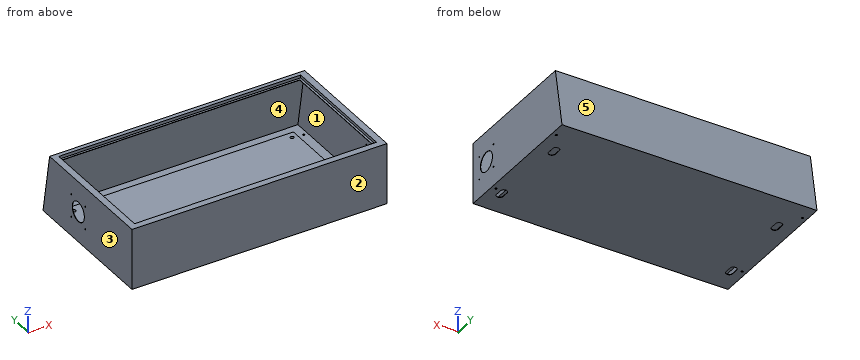
from build123d import *

# Parameters (mm, degrees)
SKETCH_1_W          = 1170
SKETCH_1_H          = 663
EXTRUDE_1_DEPTH     = 280
SKETCH_2_W          = 1110
SKETCH_2_H          = 564.628445402
CUT_EXTRUDE_1_DEPTH = 13.5
SKETCH_4_W          = 1090
SKETCH_4_H          = 544.628445402
CUT_EXTRUDE_2_DEPTH = 1.5
SHELL_START         = -583.5
SHELL_1_DEPTH       = 1167
SHELL_1_2_OUTLINE_W = 567.628445402
SHELL_1_2_OUTLINE_H = 13.5
SHELL_1_2_DEPTH     = 27
SHELL_START_2       = 556.5
SHELL_1_3_OUTLINE_W = 567.628445402
SHELL_1_3_OUTLINE_H = 13.5
SHELL_1_3_DEPTH     = 27
CUT_EXTRUDE_3_REACH = 730.366
SKETCH_5_R          = 4.5
CUT_EXTRUDE_4_REACH = 1249.875
SKETCH_6_R          = 45
SKETCH_6_R_2        = 2.75
CUT_EXTRUDE_6_REACH = 1249.875
SKETCH_8_R          = 45
SKETCH_8_R_2        = 2.75
SKETCH_9_W          = 1050
SKETCH_9_H          = 590
EXTRUDE_2_DEPTH     = 20
SKETCH_10_R         = 8.286870523
CUT_EXTRUDE_7_DEPTH = 10


# Read off the part's stored shape, not the designer's step: 抽壳1
with BuildPart() as part:
    # 草图1 → 凸台-拉伸1 (new body)
    with BuildSketch(Plane.XY):
        Rectangle(SKETCH_1_W, SKETCH_1_H)
    extrude(amount=EXTRUDE_1_DEPTH)

    # Split Bodies 1
    split(bisect_by=Plane(origin=(0, 321.504051895, 56.689838756), x_dir=(0, -0.17364817766691376, 0.984807753012211), z_dir=(0, 0.984807753012211, 0.17364817766691376)), keep=Keep.BOTTOM)

    # 草图2 → 切除-拉伸1 (cut)
    with BuildSketch(Plane.XY.offset(280)):
        with Locations((0, -19.185777299)):
            Rectangle(SKETCH_2_W, SKETCH_2_H)
    extrude(amount=-CUT_EXTRUDE_1_DEPTH, mode=Mode.SUBTRACT)

    # 草图4 → 切除-拉伸2 (cut)
    with BuildSketch(Plane.XY.offset(266.5)):
        with Locations((0, -19.185777299)):
            Rectangle(SKETCH_4_W, SKETCH_4_H)
    extrude(amount=-CUT_EXTRUDE_2_DEPTH, mode=Mode.SUBTRACT)

    # 抽壳1 outline → 抽壳1 (cut)
    with BuildSketch(Plane.YZ.offset(SHELL_START)):
        Polygon((-330, 1.5), (329.712369611, 1.5), (280.869795955, 278.5), (264.628445402, 278.5), (264.628445402, 265), (-303, 265), (-303, 278.5), (-330, 278.5), align=None)
    extrude(amount=SHELL_1_DEPTH, mode=Mode.SUBTRACT)

    # Shell 1 2 outline → Shell 1 2 (cut)
    with BuildSketch(Plane.YZ.offset(SHELL_START)):
        with Locations((-19.185777299, 271.75)):
            Rectangle(SHELL_1_2_OUTLINE_W, SHELL_1_2_OUTLINE_H)
    extrude(amount=SHELL_1_2_DEPTH, mode=Mode.SUBTRACT)

    # Shell 1 3 outline → Shell 1 3 (cut)
    with BuildSketch(Plane.YZ.offset(SHELL_START_2)):
        with Locations((-19.185777299, 271.75)):
            Rectangle(SHELL_1_3_OUTLINE_W, SHELL_1_3_OUTLINE_H)
    extrude(amount=SHELL_1_3_DEPTH, mode=Mode.SUBTRACT)

    # 草图5 → 切除-拉伸3 (cut, up to next)
    with BuildSketch(Plane(origin=(0, 0, 0), x_dir=(-1, 0, 0), z_dir=(0, 0, -1)), mode=Mode.PRIVATE) as cut_extrude_3_sk1:
        with Locations((-565, 256.5)):
            Circle(SKETCH_5_R)
    cut_extrude_3_tool1 = extrude(cut_extrude_3_sk1.sketch, amount=-CUT_EXTRUDE_3_REACH, mode=Mode.PRIVATE) & part.part
    # 草图5 → 切除-拉伸3 (cut, up to next)
    with BuildSketch(Plane(origin=(0, 0, 0), x_dir=(-1, 0, 0), z_dir=(0, 0, -1)), mode=Mode.PRIVATE) as cut_extrude_3_sk2:
        with Locations((-565, -193.5)):
            Circle(SKETCH_5_R)
    cut_extrude_3_tool2 = extrude(cut_extrude_3_sk2.sketch, amount=-CUT_EXTRUDE_3_REACH, mode=Mode.PRIVATE) & part.part
    # 草图5 → 切除-拉伸3 (cut, up to next)
    with BuildSketch(Plane(origin=(0, 0, 0), x_dir=(-1, 0, 0), z_dir=(0, 0, -1)), mode=Mode.PRIVATE) as cut_extrude_3_sk3:
        with Locations(Location((565, 256.5, 0), (0, 0, 180))):
            Circle(SKETCH_5_R)
    cut_extrude_3_tool3 = extrude(cut_extrude_3_sk3.sketch, amount=-CUT_EXTRUDE_3_REACH, mode=Mode.PRIVATE) & part.part
    # 草图5 → 切除-拉伸3 (cut, up to next)
    with BuildSketch(Plane(origin=(0, 0, 0), x_dir=(-1, 0, 0), z_dir=(0, 0, -1)), mode=Mode.PRIVATE) as cut_extrude_3_sk4:
        with Locations(Location((565, -193.5, 0), (0, 0, 180))):
            Circle(SKETCH_5_R)
    cut_extrude_3_tool4 = extrude(cut_extrude_3_sk4.sketch, amount=-CUT_EXTRUDE_3_REACH, mode=Mode.PRIVATE) & part.part
    # 草图5 → 切除-拉伸3 (cut, up to next)
    with BuildSketch(Plane(origin=(0, 0, 0), x_dir=(-1, 0, 0), z_dir=(0, 0, -1)), mode=Mode.PRIVATE) as cut_extrude_3_sk5:
        with BuildLine():
            Line((511.5, -196.5), (511.5, -226.5))
            ThreePointArc((511.5, -226.5), (526.5, -241.5), (541.5, -226.5))
            Line((541.5, -226.5), (541.5, -196.5))
            ThreePointArc((541.5, -196.5), (526.5, -181.5), (511.5, -196.5))
        make_face()
    cut_extrude_3_tool5 = extrude(cut_extrude_3_sk5.sketch, amount=-CUT_EXTRUDE_3_REACH, mode=Mode.PRIVATE) & part.part
    # 草图5 → 切除-拉伸3 (cut, up to next)
    with BuildSketch(Plane(origin=(0, 0, 0), x_dir=(-1, 0, 0), z_dir=(0, 0, -1)), mode=Mode.PRIVATE) as cut_extrude_3_sk6:
        with BuildLine():
            Line((526.5, 167.237), (526.5, 137.237))
            ThreePointArc((526.5, 137.237), (511.5, 122.237), (496.5, 137.237))
            Line((496.5, 137.237), (496.5, 167.237))
            ThreePointArc((496.5, 167.237), (511.5, 182.237), (526.5, 167.237))
        make_face()
    cut_extrude_3_tool6 = extrude(cut_extrude_3_sk6.sketch, amount=-CUT_EXTRUDE_3_REACH, mode=Mode.PRIVATE) & part.part
    # 草图5 → 切除-拉伸3 (cut, up to next)
    with BuildSketch(Plane(origin=(0, 0, 0), x_dir=(-1, 0, 0), z_dir=(0, 0, -1)), mode=Mode.PRIVATE) as cut_extrude_3_sk7:
        with BuildLine():
            Line((-541.5, -196.5), (-541.5, -226.5))
            ThreePointArc((-541.5, -226.5), (-526.5, -241.5), (-511.5, -226.5))
            Line((-511.5, -226.5), (-511.5, -196.5))
            ThreePointArc((-511.5, -196.5), (-526.5, -181.5), (-541.5, -196.5))
        make_face()
    cut_extrude_3_tool7 = extrude(cut_extrude_3_sk7.sketch, amount=-CUT_EXTRUDE_3_REACH, mode=Mode.PRIVATE) & part.part
    # 草图5 → 切除-拉伸3 (cut, up to next)
    with BuildSketch(Plane(origin=(0, 0, 0), x_dir=(-1, 0, 0), z_dir=(0, 0, -1)), mode=Mode.PRIVATE) as cut_extrude_3_sk8:
        with BuildLine():
            Line((-496.5, 167.237), (-496.5, 137.237))
            ThreePointArc((-496.5, 137.237), (-511.5, 122.237), (-526.5, 137.237))
            Line((-526.5, 137.237), (-526.5, 167.237))
            ThreePointArc((-526.5, 167.237), (-511.5, 182.237), (-496.5, 167.237))
        make_face()
    cut_extrude_3_tool8 = extrude(cut_extrude_3_sk8.sketch, amount=-CUT_EXTRUDE_3_REACH, mode=Mode.PRIVATE) & part.part
    add(cut_extrude_3_tool1.solids().sort_by_distance((565, 256.5, 0))[0], mode=Mode.SUBTRACT)
    add(cut_extrude_3_tool2.solids().sort_by_distance((565, -193.5, 0))[0], mode=Mode.SUBTRACT)
    add(cut_extrude_3_tool3.solids().sort_by_distance((-565, 256.5, 0))[0], mode=Mode.SUBTRACT)
    add(cut_extrude_3_tool4.solids().sort_by_distance((-565, -193.5, 0))[0], mode=Mode.SUBTRACT)
    add(cut_extrude_3_tool5.solids().sort_by_distance((-526.5, -211.5, 0))[0], mode=Mode.SUBTRACT)
    add(cut_extrude_3_tool6.solids().sort_by_distance((-511.5, 152.237, 0))[0], mode=Mode.SUBTRACT)
    add(cut_extrude_3_tool7.solids().sort_by_distance((526.5, -211.5, 0))[0], mode=Mode.SUBTRACT)
    add(cut_extrude_3_tool8.solids().sort_by_distance((511.5, 152.237, 0))[0], mode=Mode.SUBTRACT)

    # 草图6 → 切除-拉伸4 (cut, up to next)
    with BuildSketch(Plane(origin=(585, 0, 0), x_dir=(0, 0, -1), z_dir=(1, 0, 0)), mode=Mode.PRIVATE) as cut_extrude_4_sk1:
        with Locations((-140, -231.5)):
            Circle(SKETCH_6_R)
    cut_extrude_4_tool1 = extrude(cut_extrude_4_sk1.sketch, amount=-CUT_EXTRUDE_4_REACH, mode=Mode.PRIVATE) & part.part
    # 草图6 → 切除-拉伸4 (cut, up to next)
    with BuildSketch(Plane(origin=(585, 0, 0), x_dir=(0, 0, -1), z_dir=(1, 0, 0)), mode=Mode.PRIVATE) as cut_extrude_4_sk2:
        with Locations((-87.5, -179)):
            Circle(SKETCH_6_R_2)
    cut_extrude_4_tool2 = extrude(cut_extrude_4_sk2.sketch, amount=-CUT_EXTRUDE_4_REACH, mode=Mode.PRIVATE) & part.part
    # 草图6 → 切除-拉伸4 (cut, up to next)
    with BuildSketch(Plane(origin=(585, 0, 0), x_dir=(0, 0, -1), z_dir=(1, 0, 0)), mode=Mode.PRIVATE) as cut_extrude_4_sk3:
        with Locations(Location((-192.5, -179, 0), (0, 0, 180))):
            Circle(SKETCH_6_R_2)
    cut_extrude_4_tool3 = extrude(cut_extrude_4_sk3.sketch, amount=-CUT_EXTRUDE_4_REACH, mode=Mode.PRIVATE) & part.part
    # 草图6 → 切除-拉伸4 (cut, up to next)
    with BuildSketch(Plane(origin=(585, 0, 0), x_dir=(0, 0, -1), z_dir=(1, 0, 0)), mode=Mode.PRIVATE) as cut_extrude_4_sk4:
        with Locations((-192.5, -284)):
            Circle(SKETCH_6_R_2)
    cut_extrude_4_tool4 = extrude(cut_extrude_4_sk4.sketch, amount=-CUT_EXTRUDE_4_REACH, mode=Mode.PRIVATE) & part.part
    # 草图6 → 切除-拉伸4 (cut, up to next)
    with BuildSketch(Plane(origin=(585, 0, 0), x_dir=(0, 0, -1), z_dir=(1, 0, 0)), mode=Mode.PRIVATE) as cut_extrude_4_sk5:
        with Locations(Location((-87.5, -284, 0), (0, 0, 180))):
            Circle(SKETCH_6_R_2)
    cut_extrude_4_tool5 = extrude(cut_extrude_4_sk5.sketch, amount=-CUT_EXTRUDE_4_REACH, mode=Mode.PRIVATE) & part.part
    add(cut_extrude_4_tool1.solids().sort_by_distance((585, -231.5, 140))[0], mode=Mode.SUBTRACT)
    add(cut_extrude_4_tool2.solids().sort_by_distance((585, -179, 87.5))[0], mode=Mode.SUBTRACT)
    add(cut_extrude_4_tool3.solids().sort_by_distance((585, -179, 192.5))[0], mode=Mode.SUBTRACT)
    add(cut_extrude_4_tool4.solids().sort_by_distance((585, -284, 192.5))[0], mode=Mode.SUBTRACT)
    add(cut_extrude_4_tool5.solids().sort_by_distance((585, -284, 87.5))[0], mode=Mode.SUBTRACT)

    # 草图8 → 切除-拉伸6 (cut, up to next)
    with BuildSketch(Plane.ZY.offset(585), mode=Mode.PRIVATE) as cut_extrude_6_sk1:
        with Locations((140, 68.5)):
            Circle(SKETCH_8_R)
    cut_extrude_6_tool1 = extrude(cut_extrude_6_sk1.sketch, amount=-CUT_EXTRUDE_6_REACH, mode=Mode.PRIVATE) & part.part
    # 草图8 → 切除-拉伸6 (cut, up to next)
    with BuildSketch(Plane.ZY.offset(585), mode=Mode.PRIVATE) as cut_extrude_6_sk2:
        with Locations((192.5, 16)):
            Circle(SKETCH_8_R_2)
    cut_extrude_6_tool2 = extrude(cut_extrude_6_sk2.sketch, amount=-CUT_EXTRUDE_6_REACH, mode=Mode.PRIVATE) & part.part
    # 草图8 → 切除-拉伸6 (cut, up to next)
    with BuildSketch(Plane.ZY.offset(585), mode=Mode.PRIVATE) as cut_extrude_6_sk3:
        with Locations((87.5, 16)):
            Circle(SKETCH_8_R_2)
    cut_extrude_6_tool3 = extrude(cut_extrude_6_sk3.sketch, amount=-CUT_EXTRUDE_6_REACH, mode=Mode.PRIVATE) & part.part
    # 草图8 → 切除-拉伸6 (cut, up to next)
    with BuildSketch(Plane.ZY.offset(585), mode=Mode.PRIVATE) as cut_extrude_6_sk4:
        with Locations((87.5, 121)):
            Circle(SKETCH_8_R_2)
    cut_extrude_6_tool4 = extrude(cut_extrude_6_sk4.sketch, amount=-CUT_EXTRUDE_6_REACH, mode=Mode.PRIVATE) & part.part
    # 草图8 → 切除-拉伸6 (cut, up to next)
    with BuildSketch(Plane.ZY.offset(585), mode=Mode.PRIVATE) as cut_extrude_6_sk5:
        with Locations((192.5, 121)):
            Circle(SKETCH_8_R_2)
    cut_extrude_6_tool5 = extrude(cut_extrude_6_sk5.sketch, amount=-CUT_EXTRUDE_6_REACH, mode=Mode.PRIVATE) & part.part
    add(cut_extrude_6_tool1.solids().sort_by_distance((-585, 68.5, 140))[0], mode=Mode.SUBTRACT)
    add(cut_extrude_6_tool2.solids().sort_by_distance((-585, 16, 192.5))[0], mode=Mode.SUBTRACT)
    add(cut_extrude_6_tool3.solids().sort_by_distance((-585, 16, 87.5))[0], mode=Mode.SUBTRACT)
    add(cut_extrude_6_tool4.solids().sort_by_distance((-585, 121, 87.5))[0], mode=Mode.SUBTRACT)
    add(cut_extrude_6_tool5.solids().sort_by_distance((-585, 121, 192.5))[0], mode=Mode.SUBTRACT)

    # 草图9 → 凸台-拉伸2 (add)
    with BuildSketch(Plane.XY.offset(1.5)):
        with Locations((0, -26.5)):
            Rectangle(SKETCH_9_W, SKETCH_9_H)
    extrude(amount=EXTRUDE_2_DEPTH)

    # 草图10 → 切除-拉伸7 (cut)
    with BuildSketch(Plane.XY.offset(21.5)):
        with Locations((-500.232706652, 237.876964373)):
            Circle(SKETCH_10_R)
        with Locations(Location((500.232706652, 237.876964373, 0), (0, 0, 180))):
            Circle(SKETCH_10_R)
        with Locations((500.232706652, -288.753501232)):
            Circle(SKETCH_10_R)
        with Locations(Location((-500.232706652, -288.753501232, 0), (0, 0, 180))):
            Circle(SKETCH_10_R)
    extrude(amount=-CUT_EXTRUDE_7_DEPTH, mode=Mode.SUBTRACT)


solid = part.part
For this review, take the finished solid that the model builds, in its own axes (mm). Face numbers are marked on the shaded views. A direction names the side the tool comes from. Round coordinates to 2 decimals unless told otherwise and drop trailing zeros. Loops run counter-clockwise (first coordinate to the right, second up) from the corner with the lowest first, then second, coordinate; pieces in that order, holes last. Notation, with made-up numbers: (-4.75, 75) - (32.25, 75) arc R20 ccw to (32.25, 99) - close; hole circle Ø4 at (17, 22). An arc over 180 degrees is marked (long way). Answer as CSV lines item,"result".
(1) Consider section B-B on x = 232.5. Give the boundary of the cut face in (y, z).
Checked values:
outline,"(-331.5, 0) - (331.5, 0) - (282.13, 280) - (263.13, 280) - (263.13, 266.5) - (253.13, 266.5) - (253.13, 265) - (264.63, 265) - (264.63, 278.5) - (280.87, 278.5) - (329.71, 1.5) - (268.5, 1.5) - (268.5, 21.5) - (-321.5, 21.5) - (-321.5, 1.5) - (-330, 1.5) - (-330, 278.5) - (-303, 278.5) - (-303, 265) - (-291.5, 265) - (-291.5, 266.5) - (-301.5, 266.5) - (-301.5, 280) - (-331.5, 280) - close"
(2) Mouldability with a two-part tool opening along Y and no side actions: class the marked faces 1, 2 and 3 as +Y half, -Y half, draft (parallel to the pull), parting line (faces both ways), or undercut.
Checked values:
face 1,"undercut"
face 2,"-Y half"
face 3,"draft"
(3) Consider section C-C on z = 56. Give the boundary of the cut face in (x, y).
Checked values:
outline,"(-585, -331.5) - (585, -331.5) - (585, 321.63) - (-585, 321.63) - close; hole (-583.5, -330) - (583.5, -330) - (583.5, 320.1) - (-583.5, 320.1) - close"
(4) Tool access review of the marked faces 4 and 5: name each direction out of +Z, -Z, +X, -X, +Y, -Y from which nothing blocks a thin tool from reaching the whole face with its end or side.
Checked values:
face 4,"none"
face 5,"+Z, +X, -X, +Y"
(5) Consider section D-D on y = 211.5. Give the boundary of the cut face in (x, z).
Checked values:
outline,"(-585, 0) - (585, 0) - (585, 280) - (555, 280) - (555, 266.5) - (545, 266.5) - (545, 265) - (556.5, 265) - (556.5, 278.5) - (583.5, 278.5) - (583.5, 1.5) - (525, 1.5) - (525, 21.5) - (-525, 21.5) - (-525, 1.5) - (-583.5, 1.5) - (-583.5, 278.5) - (-556.5, 278.5) - (-556.5, 265) - (-545, 265) - (-545, 266.5) - (-555, 266.5) - (-555, 280) - (-585, 280) - close"
(6) Consider section A-A on z = 145. Give the boundary of the cut face in (x, y), then the cut area to 3 significant figures.
Checked values:
outline,"(-585, -331.5) - (585, -331.5) - (585, -276.22) - (583.5, -276.22) - (583.5, -330) - (-583.5, -330) - (-583.5, 23.78) - (-585, 23.78) - close; (-585, 113.22) - (-583.5, 113.22) - (-583.5, 304.41) - (583.5, 304.41) - (583.5, -186.78) - (585, -186.78) - (585, 305.93) - (-585, 305.93) - close"
area,"5,170 mm2"
(7) Wall thickness on line 1 (X direction, y = 287, z = 105); line 2 (Y direction, x = 94.5, z = 19); line 3 (Z direction, x = -385, y = 257): over which ranges is each line inside the solid? List them lowest first.
Checked values:
line 1,"x = -585 to -583.5, 583.5 to 585"
line 2,"y = -331.5 to -330, -321.5 to 268.5, 326.63 to 328.15"
line 3,"z = 0 to 21.5, 265 to 266.5"
(8) Insertion check: P1, Ø5, axis at x = -106.5, z = 73.5, coming from the +Y side; P2, Ø7, axis at x = -518, y = -220, coming from the -Z side; P3, Ø21.5, axis at x = -500.23, y = -288.75, coming from the +Z side; P4, Ø10.5, axis at x = 565, y = 256.5, coming from the -Z side. Each pin has a flat end and moves straight along its axis. Give the tip position at first contact, or say it passes through.
Checked values:
P1,"stops at y = 318.98"
P2,"stops at z = 1.5"
P3,"stops at z = 266.5"
P4,"stops at z = 0"
